```python
from build123d import *

# Parameters (mm, degrees)
SKETCH_2_W          = 40
SKETCH_2_H          = 40
EXTRUDE_1_DEPTH     = 12
SKETCH_3_R          = 2.5
CUT_EXTRUDE_1_DEPTH = 58.827329179
SKETCH_4_W          = 40
SKETCH_4_H          = 34.775319462
CUT_EXTRUDE_2_DEPTH = 10
SKETCH_6_R          = 3
CUT_EXTRUDE_3_DEPTH = 10
SKETCH_7_W          = 4
SKETCH_7_H          = 4
EXTRUDE_2_DEPTH     = 2
SKETCH_7_3_W        = 4
SKETCH_7_3_H        = 4
EXTRUDE_3_DEPTH     = 5.5


with BuildPart() as part:
    # Sketch 2 → Extrude 1 (new body)
    with BuildSketch(Plane.XY):
        with Locations((20, -20)):
            Rectangle(SKETCH_2_W, SKETCH_2_H)
    extrude(amount=EXTRUDE_1_DEPTH)

    # Sketch 3 → Cut-Extrude 1 (cut, through all)
    with BuildSketch(Plane(origin=(0, 0, 0), x_dir=(1, 0, 0), z_dir=(0, 1, 0))):
        with Locations(Location((7.5, -6, 0), (0, 0, 270))):
            Circle(SKETCH_3_R)
        with Locations(Location((32.5, -6, 0), (0, 0, 270))):
            Circle(SKETCH_3_R)
    extrude(amount=-CUT_EXTRUDE_1_DEPTH, mode=Mode.SUBTRACT)

    # Sketch 4 → Cut-Extrude 2 (cut)
    with BuildSketch(Plane.XY.offset(12)):
        with Locations((20, -20.159533284)):
            Rectangle(SKETCH_4_W, SKETCH_4_H)
    extrude(amount=-CUT_EXTRUDE_2_DEPTH, mode=Mode.SUBTRACT)

    # Sketch 6 → Cut-Extrude 3 (cut)
    with BuildSketch(Plane.XZ.offset(40)):
        with Locations(Location((20, 6, 0), (0, 0, 270))):
            Circle(SKETCH_6_R)
    extrude(amount=-CUT_EXTRUDE_3_DEPTH, mode=Mode.SUBTRACT)

    # Sketch 7 → Extrude 2 (add)
    with BuildSketch(Plane.XY.offset(2)):
        with Locations((28, -6)):
            Rectangle(SKETCH_7_W, SKETCH_7_H)
    extrude(amount=EXTRUDE_2_DEPTH)

    # Sketch 7_3 → Extrude 3 (add)
    with BuildSketch(Plane.XY.offset(2)):
        with Locations((12, -6)):
            Rectangle(SKETCH_7_3_W, SKETCH_7_3_H)
    extrude(amount=EXTRUDE_3_DEPTH)


solid = part.part
```
Design review of the part built by this model. Coordinates are the model's own, in mm. A direction names the side the tool comes from. Give positions to 0.01 mm unless a question says otherwise; leave off trailing zeros. Order: outer loops, then holes, each group sorted by start corner. A loop starts at its lowest first (then second) coordinate and runs counter-clockwise, first axis right, second up. Notation, with made-up numbers: (86, 25.5) - (133, 25.5) arc R10 ccw to (133, 37.5) - close; hole circle Ø1 at (82, 48). An arc over 180 degrees is marked (long way). Use a Markdown table: item, result. Add a question column.
(1) Wall thickness on probe 1 along Y at (x, z) = (11.5, 6.5); probe 2 along X at (y, z) = (-1.2, 6); probe 3 along X at (y, z) = (-39.15, 6): over which ranges is each line inside the solid? List them lowest first. Write a range as [from, to].
(2) Add section C-C on x = 20. Give the boundary of the cut face in (y, z).
(3) Clearance check with flat-ended pins moving along their axes: P1, Ø0.6, axis at y = -6, z = 3, coming from the +X side; P2, Ø5, axis at y = -15, z = 5.5, coming from the -X side; P3, Ø8, axis at x = 5.5, y = -11.5, coming from the +Z side; P4, Ø17.5, axis at x = 29.5, y = -16, coming from the +Z side. State where each tip first meets the part, or that it passes through.
(4) Add section B-B on x = 32.5. Give the boundary of the cut face in (y, z), then the cut area to 3 significant figures.
(5) Mouldability with a two-part tool opening along X and no side actions: class faces 4 (the face through (34.61, -1.37, 7.34)), 5 (the face through (10, -6, 5)), 6 (the face through (28, -6, 4)), 7 (the face through (40, -20, 1)) as +X half, -X half, draft (parallel to the pull), parting line (faces both ways), or undercut.
(6) Add section A-A on z = 9.5. Give the boundary of the cut face in (x, y), then the cut area to 3 significant figures.
(7) Machinability: for faces 1 (the face through (20, -2.772, 7)), 2 (the face through (18.85, -38.79, 3.23)), 3 (the face through (14, -6, 5)), which of the approach directions +Z, -Z, +X, -X, +Y, -Y give a long, thin tool a straight path to every point of the face, cutting with its end or side? Answer none if there is none.
(8) Add section D-D on z = 6. Give the number of separate pieces and of enclosed holes in the cut face, then the cut area to 3 significant figures.
Report:
| question | item | result |
|---|---|---|
| 1 | probe 1 | y = [-40, -37.55], [-8, -4], [-2.77, 0] |
| 1 | probe 2 | x = [0, 5], [10, 30], [35, 40] |
| 1 | probe 3 | x = [0, 5], [10, 17], [23, 30], [35, 40] |
| 2 | outline | (-40, 0) - (0, 0) - (0, 12) - (-2.77, 12) - (-2.77, 2) - (-37.55, 2) - (-37.55, 3) - (-40, 3) - close; (-40, 9) - (-37.55, 9) - (-37.55, 12) - (-40, 12) - close |
| 3 | P1 | stops at x = 30 |
| 3 | P2 | passes through |
| 3 | P3 | stops at z = 2 |
| 3 | P4 | stops at z = 4 |
| 4 | outline | (-40, 0) - (0, 0) - (0, 3.5) - (-2.77, 3.5) - (-2.77, 2) - (-37.55, 2) - (-37.55, 3.5) - (-40, 3.5) - close; (-40, 8.5) - (-37.55, 8.5) - (-37.55, 12) - (-40, 12) - close; (-2.77, 8.5) - (0, 8.5) - (0, 12) - (-2.77, 12) - close |
| 4 | area | 106 mm² |
| 5 | face 4 | undercut |
| 5 | face 5 | -X half |
| 5 | face 6 | draft |
| 5 | face 7 | +X half |
| 6 | outline | (0, -40) - (40, -40) - (40, -37.55) - (0, -37.55) - close; (0, -2.77) - (40, -2.77) - (40, 0) - (0, 0) - close |
| 6 | area | 209 mm² |
| 7 | face 1 | +Z, +X, -X |
| 7 | face 2 | -Y |
| 7 | face 3 | +Z |
| 8 | separate pieces | 8 |
| 8 | enclosed holes | 0 |
| 8 | area | 158 mm² |
